The model under review builds one solid part; all positions refer to its coordinate system, in mm. A direction names the side the tool comes from. Coordinates: 2 decimals unless noted, no trailing zeros. Write each loop counter-clockwise with the first axis right and the second up, starting at its lowest first coordinate (ties: lowest second). Pieces come first, ordered by that corner, then holes. Notation, with made-up numbers: (14.5, 79.25) - (73.5, 79.25) arc R10 cw to (73.5, 91.25) - close; hole circle Ø11 at (-3.5, 85). An arc over 180 degrees is marked (long way). Return JSON: item names as keys, results as strings. Group by question number.
(1) For pin 1 Ø2 at (x, z) = (-20.5, 49) entering from +Y, flat-tipped, find the tip position at first contact; note if it passes through.
(2) Tool access review of faces 1 (the face through (28.45, 0.78, 6.01)), 2 (the face through (-20.43, 0.78, 39.3)): name each direction out of +Z, -Z, +X, -X, +Y, -Y from which nothing blocks a thin tool from reaching the whole face with its end or side.
(3) Draft analysis for pull direction Z (two halves, no side actions). For faces 3 (the face through (34.4, 0.33, 83.13)), 4 (the face through (-31.55, 0.78, 6.01)), 5 (the face through (-42.15, 0.78, 0.57)), state which applies: released by +Z, released by -Z, zero draft, split by the parting line, or undercut.
(4) We need section B-B on x = 30. State the section outline as (y, z) points.
(5) To check wall thickness, follow L1, parallel to X at y = 0.8, z = 6.35; L2, parallel to X at y = 0.8, z = 60.5; L3, parallel to Z at x = -15, y = 0.8. State the ranges of each line that lie inside material, in increasing order. Write a range as from..to.
(6) We need section C-C on z = 6.35. State the section outline as (x, y) points.
(7) We need section A-A on z = 48. State the section outline as (x, y) points, then the cut area to 4 significant figures.
(8) We need section D-D on y = 1.1. Give the number of separate pieces and of enclosed holes in the cut face, then the cut area to 3 significant figures.
```python
from build123d import *

# Parameters (mm, degrees)
SKETCH1_R           = 1.5875
BOSS_EXTRUDE1_DEPTH = 1.5875
CUT_EXTRUDE2_DEPTH  = 116.621246561


with BuildPart() as part:
    # Sketch1 → Boss-Extrude1 (new body)
    with BuildSketch(Plane(origin=(0, 0, 0), x_dir=(1, 0, 0), z_dir=(0, 1, 0))):
        with BuildLine():
            Line((-35, -34.427940469), (-35, -81.7))
            ThreePointArc((-35, -81.7), (-34.414213562, -83.114213562), (-33, -83.7))
            Line((-33, -83.7), (-23, -83.7))
            ThreePointArc((-23, -83.7), (-21.585786438, -83.114213562), (-21, -81.7))
            Line((-21, -81.7), (-21, -40.7))
            ThreePointArc((-21, -40.7), (-20.414213562, -39.285786438), (-19, -38.7))
            Line((-19, -38.7), (19, -38.7))
            ThreePointArc((19, -38.7), (20.414213562, -39.285786438), (21, -40.7))
            Line((21, -40.7), (21, -81.7))
            ThreePointArc((21, -81.7), (21.585786438, -83.114213562), (23, -83.7))
            Line((23, -83.7), (33, -83.7))
            ThreePointArc((33, -83.7), (34.414213562, -83.114213562), (35, -81.7))
            Line((35, -81.7), (35, -34.427940469))
            ThreePointArc((35, -34.427940469), (35.120614758, -33.743900182), (35.467911114, -33.142365249))
            Line((35.467911114, -33.142365249), (42.282088886, -25.021544408))
            ThreePointArc((42.282088886, -25.021544408), (42.629385242, -24.420009476), (42.75, -23.735969189))
            Line((42.75, -23.735969189), (42.75, -2))
            ThreePointArc((42.75, -2), (42.164213562, -0.585786438), (40.75, 0))
            Line((40.75, 0), (-40.75, 0))
            ThreePointArc((-40.75, 0), (-42.164213562, -0.585786438), (-42.75, -2))
            Line((-42.75, -2), (-42.75, -23.735969189))
            ThreePointArc((-42.75, -23.735969189), (-42.629385242, -24.420009476), (-42.282088886, -25.021544408))
            Line((-42.282088886, -25.021544408), (-35.467911114, -33.142365249))
            ThreePointArc((-35.467911114, -33.142365249), (-35.120614758, -33.743900182), (-35, -34.427940469))
        make_face()
        with Locations(Location((-30, -6.35, 0), (0, 0, 270))):
            Circle(SKETCH1_R, mode=Mode.SUBTRACT)
        with Locations(Location((30, -6.35, 0), (0, 0, 270))):
            Circle(SKETCH1_R, mode=Mode.SUBTRACT)
    extrude(amount=BOSS_EXTRUDE1_DEPTH)

    # Sketch3 → Cut-Extrude2 (cut, through all)
    with BuildSketch(Plane(origin=(37, 0, 0), x_dir=(0, 0, -1), z_dir=(1, 0, 0))):
        Polygon((-81.7, 1.5875), (-55.421699883, 1.5875), (-83.7, 0.6), (-83.7, 1.5875), align=None)
    extrude(amount=-CUT_EXTRUDE2_DEPTH, mode=Mode.SUBTRACT)


solid = part.part
```
Ans:
{
 "1": {"pin 1": "y = 1.59"},
 "2": {"face 1": "+Y, -Y", "face 2": "+Z, +Y, -Y"},
 "3": {"face 3": "released by +Z", "face 4": "undercut", "face 5": "released by -Z"},
 "4": {"outline": "(0, 0) - (1.59, 0) - (1.59, 4.76) - (0, 4.76) - close; (0, 7.94) - (1.59, 7.94) - (1.59, 55.42) - (0.6, 83.7) - (0, 83.7) - close"},
 "5": {"L1": "-42.75..-31.59, -28.41..28.41, 31.59..42.75", "L2": "-35..-21, 21..35", "L3": "0..38.7"},
 "6": {"outline": "(-42.75, 0) - (-31.59, 0) - (-31.59, 1.59) - (-42.75, 1.59) - close; (-28.41, 0) - (28.41, 0) - (28.41, 1.59) - (-28.41, 1.59) - close; (31.59, 0) - (42.75, 0) - (42.75, 1.59) - (31.59, 1.59) - close"},
 "7": {"outline": "(-35, 0) - (-21, 0) - (-21, 1.59) - (-35, 1.59) - close; (21, 0) - (35, 0) - (35, 1.59) - (21, 1.59) - close", "area": "44.45 mm²"},
 "8": {"separate pieces": "1", "enclosed holes": "2", "area": "4,000 mm²"}
}
